Work out the finished part from the listing and answer in its coordinate system (mm). Round coordinates to 2 decimals unless told otherwise and drop trailing zeros. Write each loop counter-clockwise with the first axis right and the second up, starting at its lowest first coordinate (ties: lowest second). Pieces come first, ordered by that corner, then holes. Notation, with made-up numbers: (19, 20.25) -> (61, 20.25) arc R29 ccw to (61, 59.25) -> close; hole circle Ø9 at (58.5, 7.5). An arc over 180 degrees is marked (long way). Answer as a JSON object with one key per item and string values. Group by question number.
from build123d import *

# Parameters (mm, degrees)
SKETCH1_R           = 25.4
SKETCH1_W           = 203.2
SKETCH1_H           = 50.8
BOSS_EXTRUDE1_DEPTH = 25.4
SKETCH2_R           = 19.05
CUT_EXTRUDE1_DEPTH  = 22.86
SKETCH4_R           = 7.62
SKETCH4_R_2         = 1.500000048
CUT_EXTRUDE2_DEPTH  = 132.517069615
SKETCH3_R           = 3.175
CUT_EXTRUDE3_DEPTH  = 132.982271537


with BuildPart() as part:
    # Sketch1 → Boss-Extrude1 (new body)
    with BuildSketch(Plane.XY):
        with Locations((-101.6, 0)):
            Circle(SKETCH1_R)
        with Locations((101.6, 0)):
            Circle(SKETCH1_R)
        Rectangle(SKETCH1_W, SKETCH1_H)
    extrude(amount=BOSS_EXTRUDE1_DEPTH)

    # Sketch2 → Cut-Extrude1 (cut)
    with BuildSketch(Plane.XY):
        with Locations(Location((-101.6, 0, 0), (0, 0, 180))):
            Circle(SKETCH2_R)
    extrude(amount=CUT_EXTRUDE1_DEPTH, mode=Mode.SUBTRACT)

    # Sketch4 → Cut-Extrude2 (cut, through all)
    with BuildSketch(Plane(origin=(0, 0, 22.86), x_dir=(-1, 0, 0), z_dir=(0, 0, -1))):
        with Locations((101.6, 0)):
            Circle(SKETCH4_R)
        with Locations((101.6, 15.499999988)):
            Circle(SKETCH4_R_2)
        with Locations((115.023393748, 7.749999994)):
            Circle(SKETCH4_R_2)
        with Locations((115.023393748, -7.749999994)):
            Circle(SKETCH4_R_2)
        with Locations((101.6, -15.499999988)):
            Circle(SKETCH4_R_2)
        with Locations((88.176606252, -7.749999994)):
            Circle(SKETCH4_R_2)
        with Locations((88.176606252, 7.749999994)):
            Circle(SKETCH4_R_2)
    extrude(amount=-CUT_EXTRUDE2_DEPTH, mode=Mode.SUBTRACT)

    # Sketch3 → Cut-Extrude3 (cut, through all)
    with BuildSketch(Plane.XY.offset(25.4)):
        with Locations((101.6, 0)):
            Circle(SKETCH3_R)
    extrude(amount=-CUT_EXTRUDE3_DEPTH, mode=Mode.SUBTRACT)


solid = part.part
1) A cutting plane is placed at A-A on y = 0. Determine the outline of the cut face in (x, z) (3 decimals), plus the area to 3 significant figures.
2) Straight lines are drawn through the part: L1, parallel to Y at x = -101.6, z = 24.85; L2, parallel to Y at x = 101.6, z = 13.25 (3 decimals); L3, parallel to X at y = -6.5, z = 24. For each, find the intervals that lie inside material, in ascending order.
3) For a pull along Y with two mould halves and no side action, classify faces 1 (the face through (-110, 0, 22.86)), 2 (the face through (-1, -25.4, 13)), 3 (the face through (26, 0, 0)), 4 (the face through (-82.57, -0.84, 11.27)) as released by +Y, released by -Y, zero draft, split by the parting line, or undercut.
4) Each of these flat-tipped pins is pushed along its axis until it touches: P1, Ø3.5, axis at x = -101.6, y = -15.5, coming from the -Z side; P2, Ø3, axis at y = 7, z = 22, coming from the -X side; P3, Ø1.8, axis at x = -101.6, y = 15.5, coming from the +Z side; P4, Ø3, axis at y = -4.5, z = 15, coming from the +X side. Where does it stop, or does it pass through?
Established:
{
 "1": {"outline": "(-127, 0) -> (-120.65, 0) -> (-120.65, 22.86) -> (-109.22, 22.86) -> (-109.22, 25.4) -> (-127, 25.4) -> close; (-93.98, 22.86) -> (-82.55, 22.86) -> (-82.55, 0) -> (98.425, 0) -> (98.425, 25.4) -> (-93.98, 25.4) -> close; (104.775, 0) -> (127, 0) -> (127, 25.4) -> (104.775, 25.4) -> close", "area": "5,380 mm²"},
 "2": {"L1": "y = -25.4 to -17, -14 to -7.62, 7.62 to 14, 17 to 25.4", "L2": "y = -25.4 to -3.175, 3.175 to 25.4", "L3": "x = -126.15 to -115.85, -114.19 to -105.58, -97.62 to -89.01, -87.35 to 126.15"},
 "3": {"face 1": "undercut", "face 2": "released by -Y", "face 3": "zero draft", "face 4": "undercut"},
 "4": {"P1": "stops at z = 22.86", "P2": "stops at x = -126.4", "P3": "passes through", "P4": "stops at x = 126.82"}
}
